Verification items for the finished model (mm, model axes). Face numbers are marked on the shaded views. Give positions to 0.01 mm unless a question says otherwise; leave off trailing zeros. Write each loop counter-clockwise with the first axis right and the second up, starting at its lowest first coordinate (ties: lowest second). Pieces come first, ordered by that corner, then holes.
from build123d import *

# Parameters (mm, degrees)
SKETCH1_W           = 118.364
SKETCH1_H           = 72.39
BOSS_EXTRUDE1_DEPTH = 27.94
SKETCH2_R           = 4.318
BOSS_EXTRUDE2_DEPTH = 1.9558
BOSS_EXTRUDE2_TAPER = 15
FILLET1_R           = 15.24
BOSS_EXTRUDE3_DEPTH = 1.27
CUT_EXTRUDE1_DEPTH  = 4.318
SKETCH13_W          = 72.644
SKETCH13_H          = 13.208
SKETCH13_W_2        = 9.3472
SKETCH13_H_2        = 11.43
CUT_EXTRUDE2_DEPTH  = 0.635


with BuildPart() as part:
    # Sketch1 → Boss-Extrude1 (new body)
    with BuildSketch(Plane.XY):
        Rectangle(SKETCH1_W, SKETCH1_H)
    extrude(amount=BOSS_EXTRUDE1_DEPTH)

    # Sketch2 → Boss-Extrude2 (add)
    with BuildSketch(Plane(origin=(0, 0, 0), x_dir=(-1, 0, 0), z_dir=(0, 0, -1))):
        with Locations((-43.434, 21.717)):
            Circle(SKETCH2_R)
        with Locations((-43.434, -21.717)):
            Circle(SKETCH2_R)
        with Locations((43.434, -21.717)):
            Circle(SKETCH2_R)
        with Locations((43.434, 21.717)):
            Circle(SKETCH2_R)
    extrude(amount=BOSS_EXTRUDE2_DEPTH, taper=BOSS_EXTRUDE2_TAPER)

    # Fillet1
    fillet1_edges = [part.edges().sort_by_distance(p)[0] for p in [
        (-59.182, 36.195, 13.97),
        (59.182, 36.195, 13.97),
        (59.182, -36.195, 13.97),
        (-59.182, -36.195, 13.97),
    ]]
    fillet(fillet1_edges, radius=FILLET1_R)

    # Cut-Sweep1: sweep along a path in Sketch4
    with BuildLine(Plane.XY.offset(27.94)) as cut_sweep1_path:
        Line((43.942, 36.195), (-43.942, 36.195))
        ThreePointArc((-43.942, 36.195), (-54.718307345, 31.731307345), (-59.182, 20.955))
        Line((-59.182, 20.955), (-59.182, -20.955))
        ThreePointArc((-59.182, -20.955), (-54.718307345, -31.731307345), (-43.942, -36.195))
        Line((-43.942, -36.195), (43.942, -36.195))
        ThreePointArc((43.942, -36.195), (54.718307345, -31.731307345), (59.182, -20.955))
        Line((59.182, -20.955), (59.182, 20.955))
        ThreePointArc((59.182, 20.955), (54.718307345, 31.731307345), (43.942, 36.195))
    # Sketch3 → Cut-Sweep1 (sweep, cut)
    with BuildSketch(Plane(origin=(0, 0, 0), x_dir=(0, 0, -1), z_dir=(1, 0, 0))):
        Polygon((-23.495, 36.195), (-27.94, 29.591), (-27.94, 36.195), align=None)
        Polygon((0, 36.195), (0, 29.591), (-3.175, 34.417), (-3.175, 36.195), align=None)
    sweep(path=cut_sweep1_path.line, mode=Mode.SUBTRACT)

    # Sketch11 → Boss-Extrude3 (add)
    with BuildSketch(Plane(origin=(0, 0, 0), x_dir=(-1, 0, 0), z_dir=(0, 0, -1))):
        with BuildLine():
            Line((-26.67, 6.858), (-26.67, -6.858))
            ThreePointArc((-26.67, -6.858), (-32.512, -12.7), (-38.354, -6.858))
            Line((-38.354, -6.858), (-38.354, 6.858))
            ThreePointArc((-38.354, 6.858), (-32.512, 12.7), (-26.67, 6.858))
        make_face()
        with BuildLine():
            Line((26.67, 6.858), (26.67, -6.858))
            ThreePointArc((26.67, -6.858), (32.512, -12.7), (38.354, -6.858))
            Line((38.354, -6.858), (38.354, 6.858))
            ThreePointArc((38.354, 6.858), (32.512, 12.7), (26.67, 6.858))
        make_face()
    extrude(amount=BOSS_EXTRUDE3_DEPTH)

    # Sketch12 → Cut-Extrude1 (cut)
    with BuildSketch(Plane(origin=(0, 0, -1.27), x_dir=(-1, 0, 0), z_dir=(0, 0, -1))):
        with BuildLine():
            Line((-35.052, 6.858), (-35.052, 2.839806331))
            ThreePointArc((-35.052, 2.839806331), (-36.322, 0), (-35.052, -2.839806331))
            Line((-35.052, -2.839806331), (-35.052, -6.858))
            ThreePointArc((-35.052, -6.858), (-32.512, -9.398), (-29.972, -6.858))
            Line((-29.972, -6.858), (-29.972, -2.839806331))
            ThreePointArc((-29.972, -2.839806331), (-28.702, 0), (-29.972, 2.839806331))
            Line((-29.972, 2.839806331), (-29.972, 6.858))
            ThreePointArc((-29.972, 6.858), (-32.512, 9.398), (-35.052, 6.858))
        make_face()
        with BuildLine():
            Line((29.972, 2.839806331), (29.972, 6.858))
            ThreePointArc((29.972, 6.858), (32.512, 9.398), (35.052, 6.858))
            Line((35.052, 6.858), (35.052, 2.839806331))
            ThreePointArc((35.052, 2.839806331), (36.322, 0), (35.052, -2.839806331))
            Line((35.052, -2.839806331), (35.052, -6.858))
            ThreePointArc((35.052, -6.858), (32.512, -9.398), (29.972, -6.858))
            Line((29.972, -6.858), (29.972, -2.839806331))
            ThreePointArc((29.972, -2.839806331), (28.702, 0), (29.972, 2.839806331))
        make_face()
    extrude(amount=-CUT_EXTRUDE1_DEPTH, mode=Mode.SUBTRACT)

    # Sketch13 → Cut-Extrude2 (cut)
    with BuildSketch(Plane.XZ.offset(36.195)):
        with Locations((-6.4135, 14.5542)):
            Rectangle(SKETCH13_W, SKETCH13_H)
        with Locations((38.0619, 13.6652)):
            Rectangle(SKETCH13_W_2, SKETCH13_H_2)
    extrude(amount=-CUT_EXTRUDE2_DEPTH, mode=Mode.SUBTRACT)


solid = part.part
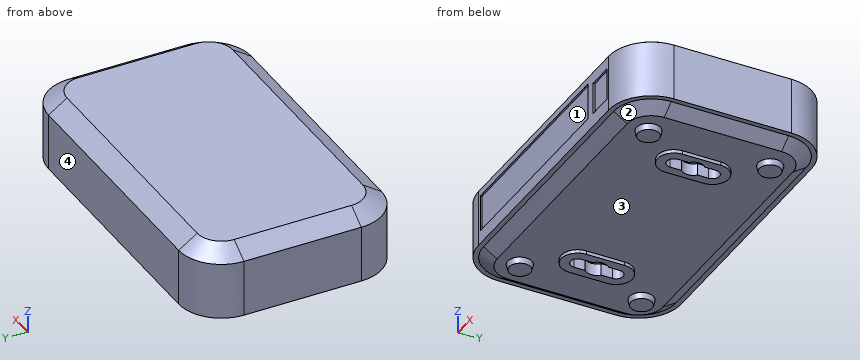
Item 1: Sectioned sample at D-D on y = -15.5. Record the cut outline in (x, z) (3 decimals).
Answer key:
outline: (-59.182, 3.175) - (-57.404, 3.175) - (-52.578, 0) - (52.578, 0) - (57.404, 3.175) - (59.182, 3.175) - (59.182, 23.495) - (52.578, 27.94) - (-52.578, 27.94) - (-59.182, 23.495) - close
Item 2: Scan lines: line 1 along Z through (x, y) = (33, 23); line 2 along Y through (x, z) = (-18, 15) (3 decimals); line 3 along X through (y, z) = (33.5, 9.5). Record each from-to range of solid material in increasing order.
Answer key:
line 1: z = 0 to 27.94
line 2: y = -35.56 to 36.195
line 3: x = -52.6 to 52.6
Item 3: Sectioned sample at B-B on z = 18. Record the cut outline in (x, y) (1 decimal).
Answer key:
outline: (-59.2, -21) arc R15.2 ccw to (-43.9, -36.2) - (-42.7, -36.2) - (-42.7, -35.6) - (29.9, -35.6) - (29.9, -36.2) - (33.4, -36.2) - (33.4, -35.6) - (42.7, -35.6) - (42.7, -36.2) - (43.9, -36.2) arc R15.2 ccw to (59.2, -21) - (59.2, 21) arc R15.2 ccw to (43.9, 36.2) - (-43.9, 36.2) arc R15.2 ccw to (-59.2, 21) - close
Item 4: Release check for a two-part mould opening along X. For the marked faces 1, 2, 3 and 4 record: released by +X, released by -X, zero draft, split by the parting line, or undercut.
Answer key:
face 1: undercut
face 2: released by +X
face 3: undercut
face 4: zero draft
Item 5: Depth check by flat-ended pin: pin 1 (1.2 mm diameter, centred on y = -5.5, z = 1, fed in from +X); pin 2 (3 mm diameter, centred on y = -4.5, z = 0, fed in from +X); pin 3 (1.2 mm diameter, centred on y = 4.5, z = 0.5, fed in from -X). Enter the tip coordinate at first touch or a pass-through.
Answer key:
pin 1: stops at x = 55.01
pin 2: stops at x = 54.86
pin 3: stops at x = -54.25
Item 6: Sectioned sample at C-C on x = -11.5. Record the cut outline in (y, z) (3 decimals), then the cut area to 3 significant figures.
Answer key:
outline: (-36.195, 3.175) - (-34.417, 3.175) - (-29.591, 0) - (29.591, 0) - (34.417, 3.175) - (36.195, 3.175) - (36.195, 23.495) - (29.591, 27.94) - (-29.591, 27.94) - (-36.195, 23.495) - (-36.195, 21.158) - (-35.56, 21.158) - (-35.56, 7.95) - (-36.195, 7.95) - close
area: 1,960 mm2
Item 7: Sectioned sample at A-A on y = 4. Record the cut outline in (x, z) (3 decimals).
Answer key:
outline: (-59.182, 3.175) - (-57.404, 3.175) - (-52.578, 0) - (-38.354, 0) - (-38.354, -1.27) - (-35.052, -1.27) - (-35.052, 3.048) - (-29.972, 3.048) - (-29.972, -1.27) - (-26.67, -1.27) - (-26.67, 0) - (26.67, 0) - (26.67, -1.27) - (29.972, -1.27) - (29.972, 3.048) - (35.052, 3.048) - (35.052, -1.27) - (38.354, -1.27) - (38.354, 0) - (52.578, 0) - (57.404, 3.175) - (59.182, 3.175) - (59.182, 23.495) - (52.578, 27.94) - (-52.578, 27.94) - (-59.182, 23.495) - close
